Build history of the part. All positions in model axes, mm. A direction names the side the tool comes from. Round coordinates to 2 decimals unless told otherwise and drop trailing zeros. Loops run counter-clockwise (first coordinate to the right, second up) from the corner with the lowest first, then second, coordinate; pieces in that order, holes last. Notation, with made-up numbers: (-8, 34) - (23, 34) arc R22 ccw to (23, 43) - close; hole circle Ø2 at (25.25, 24.5). An arc over 180 degrees is marked (long way). Use a Markdown table: item, result.
from build123d import *

# Parameters (mm, degrees)
F0_R     = 76.2
F0_R_2   = 4.7625
F1_DEPTH = 25.4


with BuildPart() as f1:
    # F0 (on Right) → F1 (new body)
    with BuildSketch(Plane.YZ):
        Circle(F0_R)
        with BuildLine():
            ThreePointArc((11.794017, 62.395121), (48.893609, 40.517465), (63.5, 0))
            ThreePointArc((63.5, 0), (48.893609, -40.517465), (11.794017, -62.395121))
            ThreePointArc((11.794017, -62.395121), (0, -63.5), (-11.794017, -62.395121))
            ThreePointArc((-11.794017, -62.395121), (-63.5, 0), (-11.794017, 62.395121))
            ThreePointArc((-11.794017, 62.395121), (0, 63.5), (11.794017, 62.395121))
        make_face(mode=Mode.SUBTRACT)
        with BuildLine():
            Line((2.358803, 12.479024), (11.794017, 62.395121))
            ThreePointArc((11.794017, 62.395121), (0, 63.5), (-11.794017, 62.395121))
            Line((-11.794017, 62.395121), (-2.358803, 12.479024))
            ThreePointArc((-2.358803, 12.479024), (0, 12.7), (2.358803, 12.479024))
        make_face()
        with BuildLine():
            ThreePointArc((12.7, 0), (9.778722, 8.103493), (2.358803, 12.479024))
            ThreePointArc((2.358803, 12.479024), (0, 12.7), (-2.358803, 12.479024))
            ThreePointArc((-2.358803, 12.479024), (-12.7, 0), (-2.358803, -12.479024))
            ThreePointArc((-2.358803, -12.479024), (0, -12.7), (2.358803, -12.479024))
            ThreePointArc((2.358803, -12.479024), (9.778722, -8.103493), (12.7, 0))
        make_face()
        Circle(F0_R_2, mode=Mode.SUBTRACT)
        with BuildLine():
            ThreePointArc((-11.794017, -62.395121), (0, -63.5), (11.794017, -62.395121))
            Line((11.794017, -62.395121), (2.358803, -12.479024))
            ThreePointArc((2.358803, -12.479024), (0, -12.7), (-2.358803, -12.479024))
            Line((-2.358803, -12.479024), (-11.794017, -62.395121))
        make_face()
    extrude(amount=F1_DEPTH)


solid = f1.part
Q1. Cut at C-C, the plane z = -19. List the corners of the cut face in (x, y), plus the area to 3 significant figures.
Results found:
| item | result |
|---|---|
| outline | (0, -73.79) - (25.4, -73.79) - (25.4, -60.59) - (0, -60.59) - close; (0, -3.59) - (25.4, -3.59) - (25.4, 3.59) - (0, 3.59) - close; (0, 60.59) - (25.4, 60.59) - (25.4, 73.79) - (0, 73.79) - close |
| area | 853 mm2 |
Q2. Drop flat-ended pins along their axis: pin 1 (8 mm diameter, centred on x = 9.5, y = -53, fed in from +Z); pin 2 (1 mm diameter, centred on x = 5, y = -0.5, fed in from +Z); pin 3 (5.5 mm diameter, centred on y = 0, z = 0, fed in from +X); pin 4 (12 mm diameter, centred on x = 8.5, y = 58.5, fed in from -Z). Give the stop position or say it passes through.
Results found:
| item | result |
|---|---|
| pin 1 | stops at z = 58.36 |
| pin 2 | stops at z = 76.2 |
| pin 3 | passes through |
| pin 4 | stops at z = -55.23 |
Q3. Cut at A-A, the plane x = 6.5. List the corners of the cut face in (y, z) (1 decimal), plus the area to 3 significant figures.
Results found:
| item | result |
|---|---|
| outline | circle Ø152.4 at (0, 0); hole (-11.8, -62.4) - (-2.4, -12.5) arc R12.7 cw to (-2.4, 12.5) - (-11.8, 62.4) arc R63.5 ccw to start; hole circle Ø9.5 at (0, 0); hole (2.4, -12.5) - (11.8, -62.4) arc R63.5 ccw to (11.8, 62.4) - (2.4, 12.5) arc R12.7 cw to (12.7, 0) arc R12.7 cw to start |
| area | 7,460 mm2 |
Q4. Cut at D-D, the plane z = -47. List the corners of the cut face in (x, y).
Results found:
| item | result |
|---|---|
| outline | (0, -59.98) - (25.4, -59.98) - (25.4, -42.7) - (0, -42.7) - close; (0, -8.88) - (25.4, -8.88) - (25.4, 8.88) - (0, 8.88) - close; (0, 42.7) - (25.4, 42.7) - (25.4, 59.98) - (0, 59.98) - close |
Q5. Cut at B-B, the plane y = 0. List the corners of the cut face in (x, z).
Results found:
| item | result |
|---|---|
| outline | (0, -76.2) - (25.4, -76.2) - (25.4, -4.76) - (0, -4.76) - close; (0, 4.76) - (25.4, 4.76) - (25.4, 76.2) - (0, 76.2) - close |
Q6. Which spindle directions (+Z, -Z, +X, -X, +Y, -Y) get a long thin tool onto all of the face, cutting with end or side? Do faces 1 (the face through (0, 5, 0)), 2 (the face through (12.522, -7.142, 37.786)). Say none if no direction does.
Results found:
| item | result |
|---|---|
| face 1 | +Z, -Z, -X, +Y, -Y |
| face 2 | +X, -X |
Q7. Probe line 1 (Y direction, x = 5.75, z = -47.5); line 2 (Y direction, x = 12.75, z = 2); line 3 (Y direction, x = 18, z = -1.5). List the from-to ranges inside material, lowest first.
Results found:
| item | result |
|---|---|
| line 1 | y = -59.58 to -42.14, -8.98 to 8.98, 42.14 to 59.58 |
| line 2 | y = -76.17 to -63.47, -12.54 to -4.32, 4.32 to 12.54, 63.47 to 76.17 |
| line 3 | y = -76.19 to -63.48, -12.61 to -4.52, 4.52 to 12.61, 63.48 to 76.19 |
Q8. Pull direction Y, two halves, no side cores. Call faces 3 (the face through (12.522, 7.142, -37.786)), 4 (the face through (12.52, -63.49, -1.23)), 5 (the face through (25.4, 5, 0)), 6 (the face through (12.522, -60.47, -46.367)): pulls with the +Y half, pulls with the -Y half, needs draft (parallel to the pull), parting line crosses it, or undercut.
Results found:
| item | result |
|---|---|
| face 3 | undercut |
| face 4 | undercut |
| face 5 | needs draft |
| face 6 | parting line crosses it |
